Verification items for this drawing (mm, ordinates from the low corner). A direction names the side the tool comes from. Give positions to 0.01 mm unless a question says otherwise; leave off trailing zeros. Loops run counter-clockwise (first coordinate to the right, second up) from the corner with the lowest first, then second, coordinate; pieces in that order, holes last. Notation, with made-up numbers: (9.25, 72.25) -> (25.25, 72.25) arc R21 ccw to (25.25, 85.25) -> close; hole circle Ø9 at (88.5, 73). An arc over 180 degrees is marked (long way). Write each question's results on one line, items separated by ' | '. Start each with the question number.
1) Sectioned sample at D-D on x = 4.75. Record the cut outline in (y, z).
2) Sectioned sample at B-B on y = 6. Record the cut outline in (x, z), then the cut area to 3 significant figures.
3) Depth check by flat-ended pin: pin 1 (2 mm diameter, centred on y = 2, z = 2.5, fed in from +X); pin 2 (3 mm diameter, centred on x = 4, y = 2, fed in from -Z); pin 3 (2 mm diameter, centred on y = 1, z = 2, fed in from -X); pin 4 (1.2 mm diameter, centred on x = 2.5, z = 2, fed in from -Y). Enter the tip coordinate at first touch or a pass-through.
4) Sectioned sample at C-C on z = 2.1. Record the cut outline in (x, y), then the cut area to 3 significant figures.
5) Draft check along X on the marked faces 1, 2, 3 and 4. Enter one of: pulls with the +X half, pulls with the -X half, needs draft (parallel to the pull), parting line crosses it, or undercut.
6) Sectioned sample at A-A on x = 3.75. Record the cut outline in (y, z).
7) Scan lines: line 1 (X direction, y = 6, z = 2.6); line 2 (Y direction, x = 3.75, z = 2.5); line 3 (Z direction, x = 2.5, y = 3.5). Record each from-to range of solid material in increasing order. Write a range as from..to.
8) Set-up check for the marked faces 5, 6, 7 and 8: record each of +Z, -Z, +X, -X, +Y, -Y from which the full face is reachable in a straight line by a thin tool's end or side.
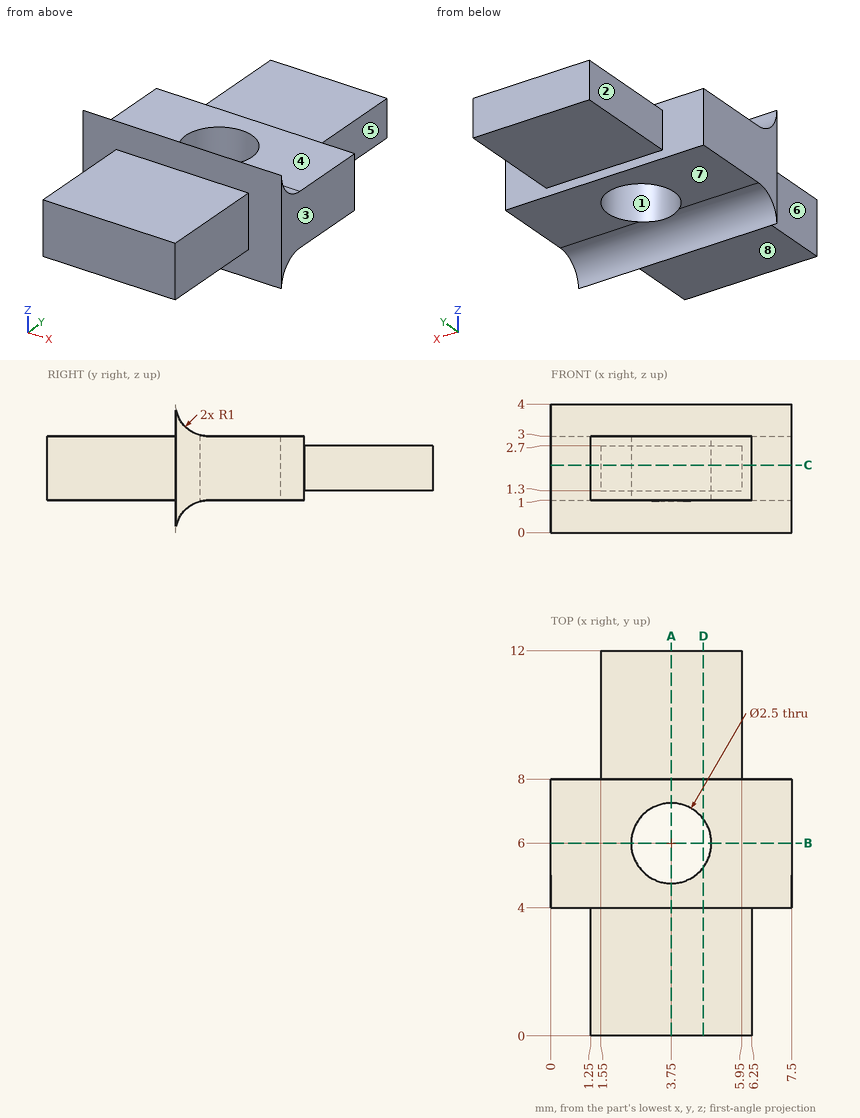
Result:
1) outline: (0, 1) -> (4, 1) -> (4, 0) arc R1 cw to (5, 1) -> (5.25, 1) -> (5.25, 3) -> (5, 3) arc R1 cw to (4, 4) -> (4, 3) -> (0, 3) -> close; (6.75, 1) -> (8, 1) -> (8, 1.3) -> (12, 1.3) -> (12, 2.7) -> (8, 2.7) -> (8, 3) -> (6.75, 3) -> close
2) outline: (0, 1) -> (2.5, 1) -> (2.5, 3) -> (0, 3) -> close; (5, 1) -> (7.5, 1) -> (7.5, 3) -> (5, 3) -> close | area: 10.0 mm^2
3) pin 1: x = 6.25 | pin 2: z = 1 | pin 3: x = 1.25 | pin 4: y = 0
4) outline: (0, 4) -> (1.25, 4) -> (1.25, 0) -> (6.25, 0) -> (6.25, 4) -> (7.5, 4) -> (7.5, 8) -> (5.95, 8) -> (5.95, 12) -> (1.55, 12) -> (1.55, 8) -> (0, 8) -> close; hole circle Ø2.5 at (3.75, 6) | area: 62.7 mm^2
5) face 1: undercut | face 2: pulls with the -X half | face 3: pulls with the +X half | face 4: needs draft
6) outline: (0, 1) -> (4, 1) -> (4, 0) arc R1 cw to (4.75, 0.97) -> (4.75, 3.03) arc R1 cw to (4, 4) -> (4, 3) -> (0, 3) -> close; (7.25, 1) -> (8, 1) -> (8, 1.3) -> (12, 1.3) -> (12, 2.7) -> (8, 2.7) -> (8, 3) -> (7.25, 3) -> close
7) line 1: 0..2.5, 5..7.5 | line 2: 0..4.75, 7.25..12 | line 3: 1..3
8) face 5: +Z, -Z, +X, +Y | face 6: +Z, -Z, -X, -Y | face 7: -Z, +X, -X, +Y | face 8: -Z, +X, -X, -Y
